The figure shows three views and two pictorial views of one solid part (mm, origin at its lowest corner). Answer the questions. A direction names the side the tool comes from. Coordinates: 2 decimals unless noted, no trailing zeros. Loops run counter-clockwise (first coordinate to the right, second up) from the corner with the lowest first, then second, coordinate; pieces in that order, holes last. Notation, with made-up numbers: M 73.25,22.25 L 97.25,22.25 A23 cw 97.25,31.25 Z; hole C -3.75,72.25 d10. An arc over 180 degrees is marked long. Answer as a JSON object with one key per item and string values. Group by question number.
1. For the marked faces 1 and 2, determine the directions among +Z, -Z, +X, -X, +Y, -Y from which every point of the face is accessible in a straight line to the end or side of a thin tool.
2. A cutting plane is placed at A-A on x = 10.5. Give the vertices of the cut face in (y, z).
3. Straight lines are drawn through the part: L1, parallel to X at y = 17.25, z = 5; L2, parallel to Y at x = 5.5, z = 1; L3, parallel to X at y = 23.5, z = 5.5. For each, find the intervals that lie inside material, in ascending order.
4. Given pin 1 (1.4 mm diameter, centred on x = 1.5, z = 5, fed in from +Y); pin 2 (6 mm diameter, centred on y = 11, z = 2, fed in from -X); pin 3 (4 mm diameter, centred on x = 10, z = 6.5, fed in from +Y); pin 4 (3 mm diameter, centred on y = 26.5, z = 5.5, fed in from +X), each flat-ended and moving along its own axis, determine where each tip first touches the part or whether it passes through.
5. A cutting plane is placed at B-B on z = 5. Give the vertices of the cut face in (x, y).
6. A cutting plane is placed at D-D on z = 2. Give the vertices of the cut face in (x, y).
7. A cutting plane is placed at C-C on y = 22. Give the vertices of the cut face in (x, z), and give its area (3 significant figures).
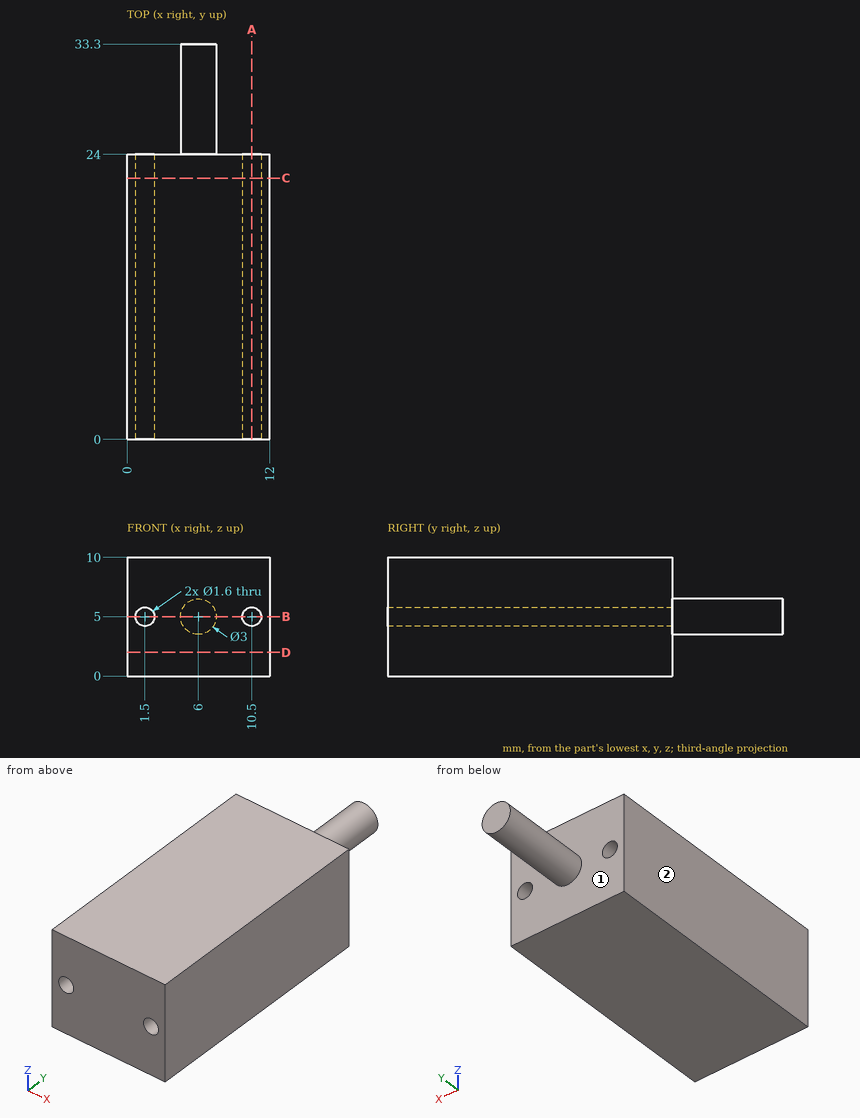
From the geometry:
{
 "1": {"face 1": "+Y", "face 2": "+Z, -Z, -X, +Y, -Y"},
 "2": {"outline": "M 0,0 L 24,0 L 24,4.2 L 0,4.2 Z; M 0,5.8 L 24,5.8 L 24,10 L 0,10 Z"},
 "3": {"L1": "x = 0 to 0.7, 2.3 to 9.7, 11.3 to 12", "L2": "y = 0 to 24", "L3": "x = 0 to 0.88, 2.12 to 9.88, 11.12 to 12"},
 "4": {"pin 1": "passes through", "pin 2": "stops at x = 0", "pin 3": "stops at y = 24", "pin 4": "stops at x = 7.5"},
 "5": {"outline": "M 0,0 L 0.7,0 L 0.7,24 L 0,24 Z; M 2.3,0 L 9.7,0 L 9.7,24 L 7.5,24 L 7.5,33.3 L 4.5,33.3 L 4.5,24 L 2.3,24 Z; M 11.3,0 L 12,0 L 12,24 L 11.3,24 Z"},
 "6": {"outline": "M 0,0 L 12,0 L 12,24 L 0,24 Z"},
 "7": {"outline": "M 0,0 L 12,0 L 12,10 L 0,10 Z; hole C 1.5,5 d1.6; hole C 10.5,5 d1.6", "area": "116 mm²"}
}
